For this review, take the finished solid that the model builds, in its own axes (mm). Give positions to 0.01 mm unless a question says otherwise; leave off trailing zeros. Write each loop counter-clockwise with the first axis right and the second up, starting at its lowest first coordinate (ties: lowest second). Pieces come first, ordered by that corner, then holes.
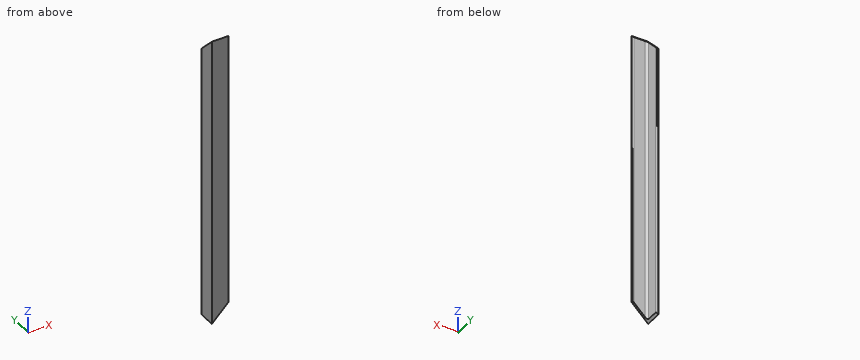
Autodesk Inventor part; units mm, degrees
ref_plane "Start Plane" through (0, 0, 0) normal (0, 0, 1) x (1, 0, 0)
ref_plane "End Plane" through (0, 0, 450) normal (0, 0, 1) x (1, 0, 0)
ref_plane "Work Plane5" through (12.7, 0, 450) normal (0, 0.7071, 0.7071) x (1, 0, 0)
ref_plane "Start Plane" through (0, 0, 0) normal (0, 0, 1) x (1, 0, 0)
ref_plane "End Plane" through (0, 0, 450) normal (0, 0, 1) x (1, 0, 0)
sketch "Sketch" plane through (0, 0, 0) normal (0, 0, 1) x (1, 0, 0)
  line L0 (25.4, 0) -> (0, 0)
  line L1 (0, 0) -> (0, 25.4)
  line L2 (0, 25.4) -> (1.651, 25.4)
  line L3 (3.175, 23.876) -> (3.175, 6.477)
  line L4 (6.477, 3.175) -> (23.876, 3.175)
  line L5 (25.4, 1.651) -> (25.4, 0)
  line L6 (0, -11.0414) -> (0, 31.5385) construction
  line L7 (-11.0414, 0) -> (31.5385, 0) construction
  arc A0 (3.175, 6.477) -> (6.477, 3.175) centre (6.477, 6.477) ccw
  arc A1 (3.175, 23.876) -> (1.651, 25.4) centre (1.651, 23.876) ccw
  arc A2 (25.4, 1.651) -> (23.876, 3.175) centre (23.876, 1.651) ccw
  line L8 (0, 40.0545) -> (0, -19.5574) construction
  line L9 (-19.5574, 0) -> (40.0545, 0) construction
  point P0 (3.175, 25.4)
  point P1 (3.175, 3.175)
  point P2 (25.4, 3.175)
  dimension "d0" = 25.4
  dimension "d1" = 25.4
  dimension "d2" = 3.175
  dimension "d3" = 3.175
  dimension "d10" = 0
  dimension "d11" = 0
  dimension "d14" = 3.302
  dimension "d15" = 1.524
extrude "Body" add sketch "Sketch" along normal up to surface (450 mm away) from surface at 0
sketch "Sketch3" plane through (0, 0, 0) normal (0, 0, 1) x (1, 0, 0)
  line L0 (0, 0) -> (10, 0)
ref_plane "Work Plane3" through (0, 0, 0) normal (0, -1, 0) x (1, 0, 0)
ref_plane "Work Plane5" through (12.7, 0, 450) normal (0, 0.7071, 0.7071) x (1, 0, 0)
split "Split2" plane through (12.7, 0, 450) removes the side toward (0, 0.7071, 0.7071)
ref_plane "Work Plane6" through (0, 12.7, 0) normal (0.7071, 0, -0.7071) x (-0.7071, 0, -0.7071)
split "Split3" plane through (0, 12.7, 0) removes the side toward (0.7071, 0, -0.7071)
sketch "Sketch4" plane through (0, 0, 0) normal (0, -1, 0) x (1, 0, 0)
  line L0 (-2, 0) -> (12, 0)
  line L1 (-2, 450) -> (12, 450)
  dimension "d17" = 450
equation "\"d0\" = G_H"
equation "\"d1\" = G_H"
equation "\"d2\" = G_T"
equation "\"d3\" = G_T"
equation "\"d14\" = G_IR"
equation "\"d15\" = G_ER"
equation "\"d4\" = G_L"
equation "\"G_H\" = 25.4"
equation "\"G_T\" = 3.175"
equation "\"G_ER\" = 1.524"
equation "\"G_IR\" = 3.302"
equation "\"G_L\" = d17"
equation "\"ex\" = 0"
equation "\"G_OFFSET_START\" = 0"
equation "\"G_OFFSET_END\" = 0"
equation "\"d13\" = G_OFFSET_END + B_L"
equation "\"B_L\" = 450"
properties part number "AISC - L 1 x 1 x 1/8 - 17.717" material "Steel, Mild"
(1) Clearance check with flat-ended pins moving along their axes: pin 1 Ø1 at (x, z) = (13.5, 365) entering from -Y; pin 2 Ø14 at (x, z) = (17, 310) entering from +Y (3 decimals); pin 3 Ø5 at (y, z) = (9.5, 59.5) entering from +X (3 decimals); pin 4 Ø1.5 at (x, y) = (12, 2.5) entering from -Z. State where each tip first meets the part, or that it passes through.
(2) For L1, parallel to X at y = 21.5, z = 246 (3 decimals); L2, parallel to X at y = 4, z = 406.5, list the stretches that pass through material, from the lowest coordinate up.
(3) We need section C-C (x = 16.75). Write out the cut boundary in (y, z) (3 decimals).
(4) We need section B-B (y = 10.25). Write out the cut boundary in (x, z) (3 decimals), and give its area (3 significant figures).
(5) We need section A-A (z = 307). Write out the cut boundary in (x, y) (3 decimals), and give its area (3 significant figures).
The answers:
1. pin 1: stops at y = 0
1. pin 2: stops at y = 3.175
1. pin 3: stops at x = 3.175
1. pin 4: stops at z = 11.25
2. L1: x = 0 to 3.175
2. L2: x = 0 to 4.29
3. outline: (0, 16.75) - (3.175, 16.75) - (3.175, 446.825) - (0, 450) - close
4. outline: (0, 0) - (3.175, 3.175) - (3.175, 439.75) - (0, 439.75) - close
4. area: 1,390 mm2
5. outline: (0, 0) - (25.4, 0) - (25.4, 1.651) arc R1.524 ccw to (23.876, 3.175) - (6.477, 3.175) arc R3.302 cw to (3.175, 6.477) - (3.175, 23.876) arc R1.524 ccw to (1.651, 25.4) - (0, 25.4) - close
5. area: 153 mm2
